```python
from build123d import *

# Parameters (mm, degrees)
SKETCH2_R = 9
SHELL1_T  = -1


with BuildPart() as part:
    # Sweep1: sweep along a path in Sketch1
    with BuildLine(Plane.XY) as sweep1_path:
        Line((-102.114386638, 38.661028062), (-102.114386638, -41.338971938))
        ThreePointArc((-102.114386638, -41.338971938), (-97.720988356, -51.945573656), (-87.114386638, -56.338971938))
        Line((-87.114386638, -56.338971938), (-27.114386638, -56.338971938))
    # Sketch2 → Sweep1 (sweep)
    with BuildSketch(Plane(origin=(0, 38.661028062, 0), x_dir=(1, 0, 0), z_dir=(0, 1, 0))):
        with Locations((-102.114386638, 0)):
            Circle(SKETCH2_R)
    sweep(path=sweep1_path.line)

    # Shell1
    shell1_openings = [part.faces().sort_by_distance(p)[0] for p in [
        (-27.114386638, -56.338971938, 0),
        (-102.114386638, 38.661028062, 0),
    ]]
    offset(amount=SHELL1_T, openings=shell1_openings, kind=Kind.INTERSECTION)


solid = part.part
```
For this review, take the finished solid that the model builds, in its own axes (mm). Coordinates: 2 decimals unless noted, no trailing zeros. Write each loop counter-clockwise with the first axis right and the second up, starting at its lowest first coordinate (ties: lowest second). Pieces come first, ordered by that corner, then holes.
(1) For pin 1 Ø1 at (y, z) = (11, 5) entering from -X; pin 2 Ø4 at (y, z) = (-44, 0.5) entering from +X; pin 3 Ø10 at (y, z) = (-16.5, -0.5) entering from +X, all flat-tipped, find the tip position at first contact; note any pin that passes through.
(2) Add section B-B on x = -82.5. Give the boundary of the cut face in (y, z), then the cut area to 3 significant figures.
(3) Wall thickness on probe 1 along X at (y, z) = (11.5, 0.5); probe 2 along Z at (x, y) = (-104.5, 20); probe 3 along Y at (x, z) = (-37, 4.5): over which ranges is each line inside the solid? List them lowest first.
(4) Add section C-C on y = -2.5. Give the boundary of the cut face in (x, z).
(5) The part is to be moulded in two halves that separate along X. For faces 1 (the face through (-94.724, -1.899, -3.064)), 2 (the face through (-93.53, -1.9, 2.7)), 3 (the face through (-56.694, -47.755, 2.703)), say which applies: +X half, -X half, draft (parallel to the pull), parting line (faces both ways), or undercut.
(6) Add section A-A on z = 0. Give the boundary of the cut face in (x, y).
(7) Add section D-D on z = 6. Give the boundary of the cut face in (x, y), then the cut area to 3 significant figures.
Answer sheet:
1. pin 1: stops at x = -109.91
1. pin 2: stops at x = -90.91
1. pin 3: stops at x = -93.11
2. outline: circle Ø18 at (-56.34, 0); hole circle Ø16 at (-56.34, 0)
2. area: 53.4 mm2
3. probe 1: x = -111.1 to -110.1, -94.13 to -93.13
3. probe 2: z = -8.68 to -7.64, 7.64 to 8.68
3. probe 3: y = -64.13 to -62.95, -49.72 to -48.54
4. outline: circle Ø18 at (-102.11, 0); hole circle Ø16 at (-102.11, 0)
5. face 1: undercut
5. face 2: parting line
5. face 3: draft
6. outline: (-111.11, -41.34) arc R24 ccw to (-87.11, -65.34) - (-27.11, -65.34) - (-27.11, -64.34) - (-87.11, -64.34) arc R23 cw to (-110.11, -41.34) - (-110.11, 38.66) - (-111.11, 38.66) - close; (-94.11, -41.34) arc R7 ccw to (-87.11, -48.34) - (-27.11, -48.34) - (-27.11, -47.34) - (-87.11, -47.34) arc R6 cw to (-93.11, -41.34) - (-93.11, 38.66) - (-94.11, 38.66) - close
7. outline: (-108.82, -41.34) arc R21.71 ccw to (-87.11, -63.05) - (-27.11, -63.05) - (-27.11, -61.63) - (-87.11, -61.63) arc R20.29 cw to (-107.41, -41.34) - (-107.41, 38.66) - (-108.82, 38.66) - close; (-96.82, -41.34) arc R9.71 ccw to (-87.11, -51.05) - (-27.11, -51.05) - (-27.11, -49.63) - (-87.11, -49.63) arc R8.29 cw to (-95.41, -41.34) - (-95.41, 38.66) - (-96.82, 38.66) - close
7. area: 463 mm2
